Check sheet for the drawn part. Datum: minimum x, y, z corner. Units: mm. Round coordinates to 2 decimals unless told otherwise and drop trailing zeros. Write each loop counter-clockwise with the first axis right and the second up, starting at its lowest first coordinate (ties: lowest second). Pieces come first, ordered by that corner, then holes. Notation, with made-up numbers: (-39.75, 21) - (-11.75, 21) arc R16 ccw to (-11.75, 27) - close; hole circle Ø5 at (29, 73.25). An arc over 180 degrees is marked (long way). Answer as a JSON object with one key per item and string values. Group by question number.
Item 1: Sectioned sample at C-C on x = 10. Record the boundary of the cut face in (y, z), plus the area to 3 significant figures.
Item 2: Sectioned sample at B-B on y = 1.6. Record the boundary of the cut face in (x, z).
Item 3: Gauge pin test, flat ends, axial feed: P1, Ø1.5, axis at x = 2, y = 1, coming from the -Z side; P2, Ø1.5, axis at y = 2, z = 45, coming from the -X side; P3, Ø1.5, axis at y = 1.5, z = 1, coming from the +X side. Record the tip position at first contact, or that the pin passes through.
Item 4: Thickness scan on line 1 (Z direction, x = 10, y = 2.3); line 2 (X direction, y = 1.45, z = 36.5); line 3 (X direction, y = 0.5, z = 16.5). Record the ranges inside material, lowest first.
Item 5: Sectioned sample at D-D on x = 14.75. Record the boundary of the cut face in (y, z), plus the area to 3 significant figures.
Item 6: Sectioned sample at A-A on z = 26.5. Record the boundary of the cut face in (x, y).
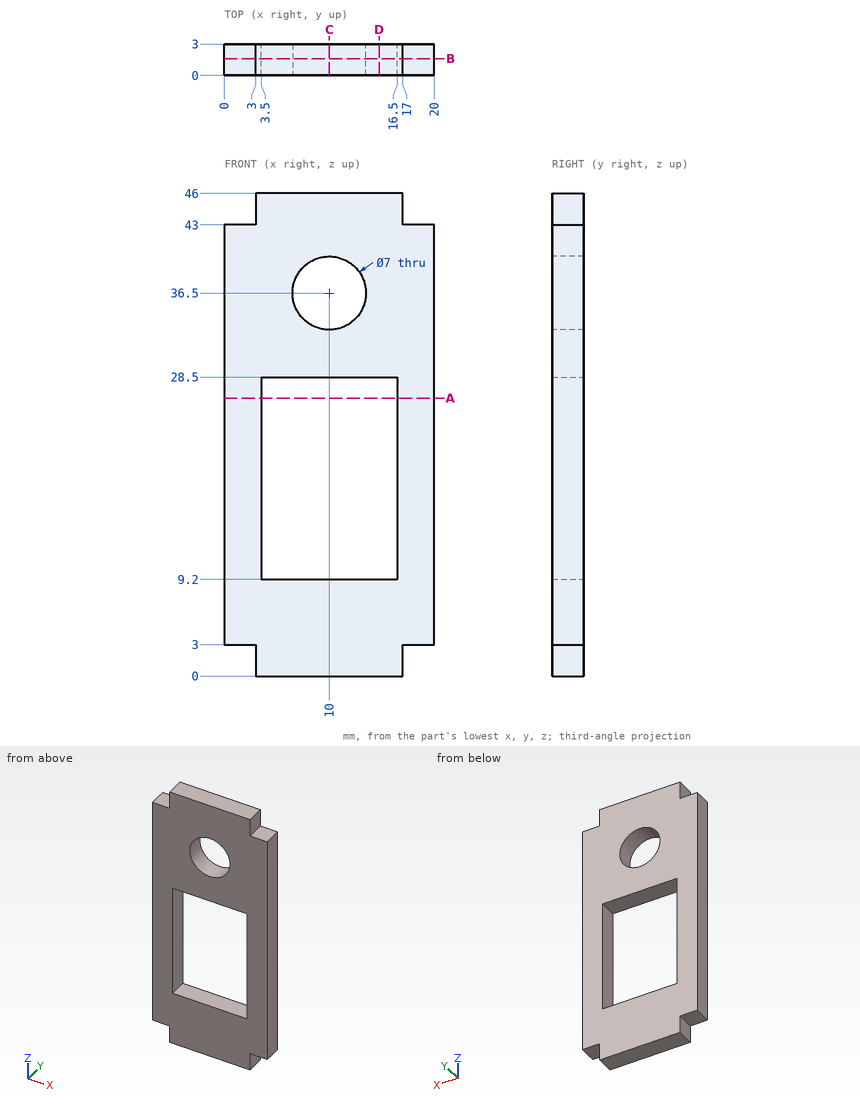
Completed:
{
 "1": {"outline": "(0, 0) - (3, 0) - (3, 9.2) - (0, 9.2) - close; (0, 28.5) - (3, 28.5) - (3, 33) - (0, 33) - close; (0, 40) - (3, 40) - (3, 46) - (0, 46) - close", "area": "59.1 mm²"},
 "2": {"outline": "(0, 3) - (3, 3) - (3, 0) - (17, 0) - (17, 3) - (20, 3) - (20, 43) - (17, 43) - (17, 46) - (3, 46) - (3, 43) - (0, 43) - close; hole (3.5, 9.2) - (16.5, 9.2) - (16.5, 28.5) - (3.5, 28.5) - close; hole circle Ø7 at (10, 36.5)"},
 "3": {"P1": "z = 3", "P2": "x = 3", "P3": "x = 17"},
 "4": {"line 1": "0 to 9.2, 28.5 to 33, 40 to 46", "line 2": "0 to 6.5, 13.5 to 20", "line 3": "0 to 3.5, 16.5 to 20"},
 "5": {"outline": "(0, 0) - (3, 0) - (3, 9.2) - (0, 9.2) - close; (0, 28.5) - (3, 28.5) - (3, 46) - (0, 46) - close", "area": "80.1 mm²"},
 "6": {"outline": "(0, 0) - (3.5, 0) - (3.5, 3) - (0, 3) - close; (16.5, 0) - (20, 0) - (20, 3) - (16.5, 3) - close"}
}
